Can you work these out from the model? Positions are in its coordinate system, mm. Face numbers are marked on the shaded views. A direction names the side the tool comes from. Round coordinates to 2 decimals unless told otherwise and drop trailing zeros. Order: outer loops, then holes, each group sorted by start corner. A loop starts at its lowest first (then second) coordinate and runs counter-clockwise, first axis right, second up. Notation, with made-up numbers: M 45,53 L 82,53 A20 ccw 82,81 Z; hole C -8.5,-31 d1. An arc over 180 degrees is marked long. Answer as CSV lines item,"result". Start each with the question number.
from build123d import *

# Parameters (mm, degrees)
F0_R     = 62.5
F0_R_2   = 12.5
F1_DEPTH = 10
F2_R     = 62.5
F3_DEPTH = 2.5


with BuildPart() as f1:
    # F0 (on Top) → F1 (new body)
    with BuildSketch(Plane.XY):
        Circle(F0_R)
        with Locations((-30, -30)):
            Circle(F0_R_2, mode=Mode.SUBTRACT)
        with Locations((0, -30)):
            Circle(F0_R_2, mode=Mode.SUBTRACT)
        with Locations((30, -30)):
            Circle(F0_R_2, mode=Mode.SUBTRACT)
        with Locations((-30, 0)):
            Circle(F0_R_2, mode=Mode.SUBTRACT)
        with Locations((-30, 30)):
            Circle(F0_R_2, mode=Mode.SUBTRACT)
        Circle(F0_R_2, mode=Mode.SUBTRACT)
        with Locations((30, 0)):
            Circle(F0_R_2, mode=Mode.SUBTRACT)
        with Locations((0, 30)):
            Circle(F0_R_2, mode=Mode.SUBTRACT)
        with Locations((30, 30)):
            Circle(F0_R_2, mode=Mode.SUBTRACT)
    extrude(amount=F1_DEPTH)

    # F2 (on Top) → F3 (join)
    with BuildSketch(Plane.XY):
        Circle(F2_R)
    extrude(amount=F3_DEPTH)


solid = f1.part
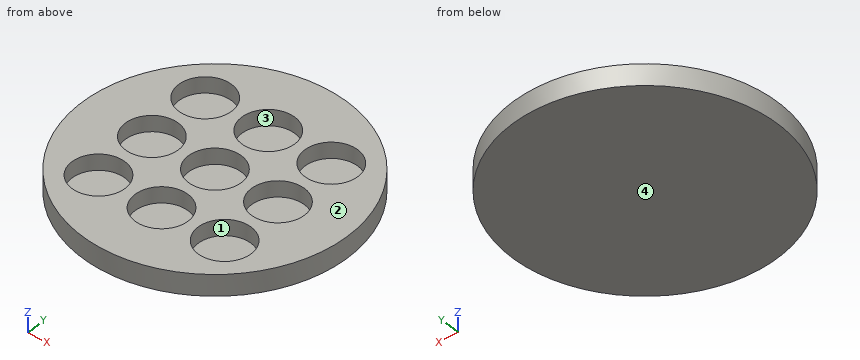
(1) I want a section at A-A on y = 0. Write out the boundary of the cut face in (x, z).
(2) I want a section at D-D on x = 48.5. Write out the boundary of the cut face in (y, z).
(3) If I drill on line 1 along Y through (x, z) = (0, 8.75); line 2 along Y through (x, z) = (-30, 4), over which ranges is the centre line in solid material (lowest first)?
(4) I'm going to push flat-ended pins straight in: P1, Ø2, axis at x = 10.5, z = 5.5, coming from the +Y side; P2, Ø22.5, axis at x = 30, y = 30, coming from the +Z side; P3, Ø5, axis at x = -46, z = 5, coming from the -Y side. Where does each tip first touch, or does it pass through?
(5) If we mould it in two halves opening along X, with no side actions, what happens to the marked faces 1 and 2? For each: +X half, -X half, draft (parallel to the pull), parting line (faces both ways), or undercut.
(6) I want a section at C-C on x = -22. Write out the boundary of the cut face in (y, z), and give its area (3 significant figures).
(7) I want a section at B-B on z = 6.5. Count the separate pieces of the cut face and the enclosed holes in it, and give its area (3 significant figures).
(8) For the marked faces 3 and 4, which set-ups out of +Z, -Z, +X, -X, +Y, -Y let a thin tool reach every point of the face, with its end or its side?
From the geometry:
1,outline,"M -62.5,0 L 62.5,0 L 62.5,10 L 42.5,10 L 42.5,2.5 L 17.5,2.5 L 17.5,10 L 12.5,10 L 12.5,2.5 L -12.5,2.5 L -12.5,10 L -17.5,10 L -17.5,2.5 L -42.5,2.5 L -42.5,10 L -62.5,10 Z"
2,outline,"M -39.42,0 L 39.42,0 L 39.42,10 L -39.42,10 Z"
3,line 1,"-62.5 to -42.5, -17.5 to -12.5, 12.5 to 17.5, 42.5 to 62.5"
3,line 2,"-54.83 to -42.5, -17.5 to -12.5, 12.5 to 17.5, 42.5 to 54.83"
4,P1,"y = 61.77"
4,P2,"z = 2.5"
4,P3,"y = -44.88"
5,face 1,"undercut"
5,face 2,"draft"
6,outline,"M -58.5,0 L 58.5,0 L 58.5,10 L 39.6,10 L 39.6,2.5 L 20.4,2.5 L 20.4,10 L 9.6,10 L 9.6,2.5 L -9.6,2.5 L -9.6,10 L -20.4,10 L -20.4,2.5 L -39.6,2.5 L -39.6,10 L -58.5,10 Z"
6,area,"738 mm²"
7,separate pieces,"1"
7,enclosed holes,"9"
7,area,"7,850 mm²"
8,face 3,"+Z"
8,face 4,"-Z, +X, -X, +Y, -Y"
